Read the model definition and answer for the solid it produces. Units are mm, in the model's axes. A direction names the side the tool comes from. Round coordinates to 2 decimals unless told otherwise and drop trailing zeros. Order: outer loops, then holes, each group sorted by start corner. A loop starts at its lowest first (then second) coordinate and runs counter-clockwise, first axis right, second up. Notation, with made-up numbers: (-8, 60) -> (34, 60) arc R17 ccw to (34, 80) -> close; hole circle Ø2 at (-25.75, -13). An arc over 180 degrees is marked (long way). One line per item, written item: value. Start each with the question number.
1. The mould has two halves that part along X. Classify faces 3 (the face through (-6.5, 0.1, -50.8)), 4 (the face through (0, -6.35, -25)), 5 (the face through (-9.525, 0, -25)): released by +X, released by -X, zero draft, split by the parting line, or undercut.
2. Section B-B (y = 1.25) is taken. Give the vertices of the cut face in (x, z) (3 decimals), then the cut area to 3 significant figures.
3. For faces 1 (the face through (6.35, 0, -25)), 2 (the face through (9.525, 0, -25)), determine the directions among +Z, -Z, +X, -X, +Y, -Y from which every point of the face is accessible in a straight line to the end or side of a thin tool.
4. Consider line 1 (X direction, y = 4.5, z = -31) (3 decimals). Determine where the line is inside the solid, lowest interval first.
5. Flat-ended cylindrical pins translate along their axes: pin 1 Ø1 at (x, y) = (4.5, 3.5) entering from -Z; pin 2 Ø8 at (x, y) = (6, 3.5) entering from +Z. Find the tip coordinate at first contact, or state that the pin passes through.
6. Section A-A (z = -25.5) is taken. Give the vertices of the cut face in (x, y) (3 decimals), then the cut area to 3 significant figures.
from build123d import *

# Parameters (mm, degrees)
SKETCH1_W           = 19.05
SKETCH1_H           = 19.05
BOSS_EXTRUDE1_DEPTH = 50.8
CUT_EXTRUDE1_REACH  = 52.8
SKETCH2_W           = 12.7
SKETCH2_H           = 12.7


with BuildPart() as part:
    # Sketch1 → Boss-Extrude1 (new body)
    with BuildSketch(Plane.XY):
        Rectangle(SKETCH1_W, SKETCH1_H)
    extrude(amount=-BOSS_EXTRUDE1_DEPTH)

    # Sketch2 → Cut-Extrude1 (cut, up to next)
    with BuildSketch(Plane.XY, mode=Mode.PRIVATE) as cut_extrude1_sk1:
        Rectangle(SKETCH2_W, SKETCH2_H)
    cut_extrude1_tool1 = extrude(cut_extrude1_sk1.sketch, amount=-CUT_EXTRUDE1_REACH, mode=Mode.PRIVATE) & part.part
    add(cut_extrude1_tool1.solids().sort_by_distance((0, 0, 0))[0], mode=Mode.SUBTRACT)


solid = part.part
Answer:
1. face 3: zero draft
1. face 4: undercut
1. face 5: released by -X
2. outline: (-9.525, -50.8) -> (-6.35, -50.8) -> (-6.35, 0) -> (-9.525, 0) -> close; (6.35, -50.8) -> (9.525, -50.8) -> (9.525, 0) -> (6.35, 0) -> close
2. area: 323 mm^2
3. face 1: +Z, -Z
3. face 2: +Z, -Z, +X, +Y, -Y
4. line 1: -9.525 to -6.35, 6.35 to 9.525
5. pin 1: through
5. pin 2: z = 0
6. outline: (-9.525, -9.525) -> (9.525, -9.525) -> (9.525, 9.525) -> (-9.525, 9.525) -> close; hole (-6.35, -6.35) -> (6.35, -6.35) -> (6.35, 6.35) -> (-6.35, 6.35) -> close
6. area: 202 mm^2
